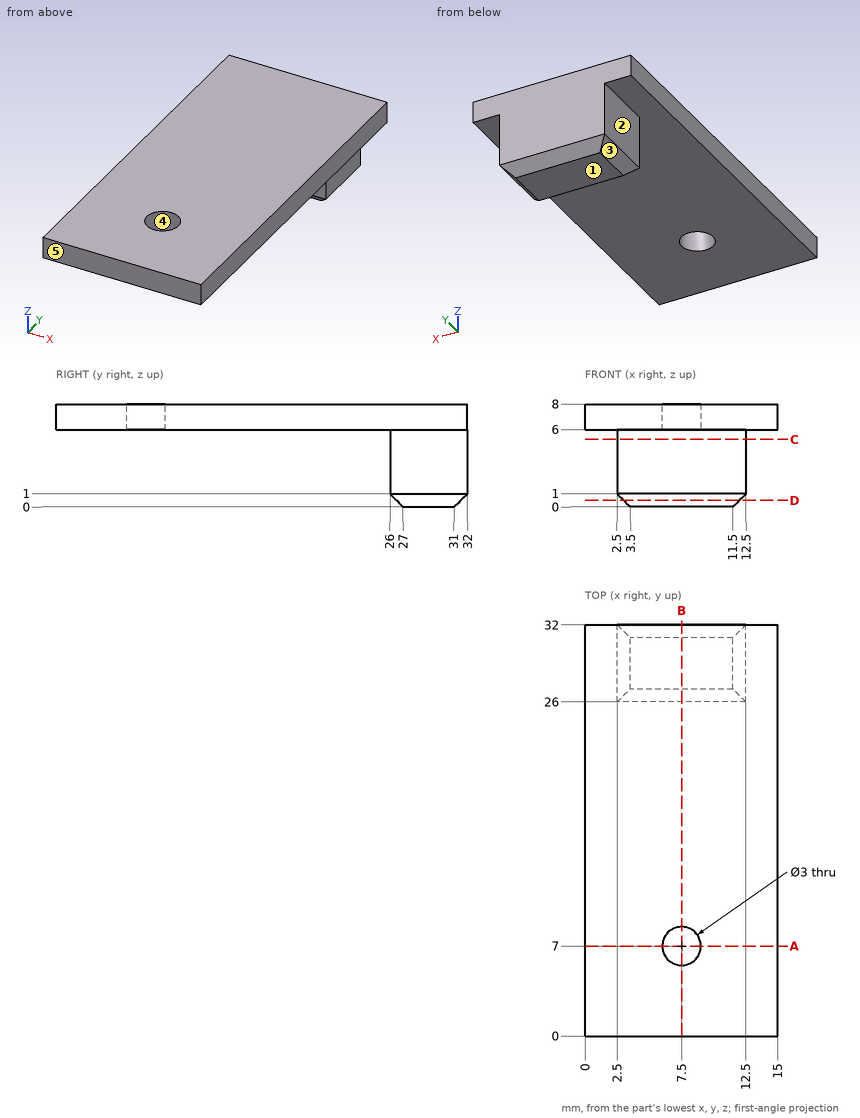
Here's the drawing with two shaded views (mm, measured from the low corner). I have some questions. A direction names the side the tool comes from. Give positions to 0.01 mm unless a question says otherwise; leave off trailing zeros. Write each loop counter-clockwise with the first axis right and the second up, starting at its lowest first coordinate (ties: lowest second). Pieces come first, ordered by that corner, then holes. Notation, with made-up numbers: (28.25, 50.25) - (47.25, 50.25) arc R28 ccw to (47.25, 70.25) - close; hole circle Ø5 at (-39.75, 50.25). An arc over 180 degrees is marked (long way). One line per item, written item: value. Start each with the question number.
Item 1: Please list where these lines run through material, in increasing order: line 1 (Y direction, x = 7.5, z = 6.85); line 2 (Y direction, x = 10.5, z = 1.5); line 3 (Z direction, x = 5.5, y = 10). Write a range as from..to.
Item 2: Which directions (+Z, -Z, +X, -X, +Y, -Y) give clear straight access to the entire face, cutting with the end or side of a thin tool? Please do the marked faces 1 and 2.
Item 3: Imagine slicing it at B-B, the plane x = 7.5. List the corners of the cut face in (y, z) for me, and give its area (3 significant figures).
Item 4: If we mould it in two halves opening along X, with no side actions, what happens to the marked faces 3, 4 and 5? For each: +X half, -X half, draft (parallel to the pull), parting line (faces both ways), or undercut.
Item 5: Imagine slicing it at A-A, the plane y = 7. List the corners of the cut face in (x, z) for me.
Item 6: Imagine slicing it at C-C, the plane z = 5.25. List the corners of the cut face in (x, y) for me.
Item 7: Imagine slicing it at D-D, the plane z = 0.5. List the corners of the cut face in (x, y) for me.
Item 8: I'm going to push flat-ended pins straight in: pin 1 (7.5 mm diameter, centred on x = 9, y = 17.5, fed in from -Z); pin 2 (1.5 mm diameter, centred on x = 8, z = 4, fed in from -Y); pin 3 (2 mm diameter, centred on y = 25.5, z = 2, fed in from +X). Where does each tip first touch, or does it pass through?
Geometry says:
1. line 1: 0..5.5, 8.5..32
1. line 2: 26..32
1. line 3: 6..8
2. face 1: -Z, +X, -X, +Y, -Y
2. face 2: -Z, -X, +Y, -Y
3. outline: (0, 6) - (5.5, 6) - (5.5, 8) - (0, 8) - close; (8.5, 6) - (26, 6) - (26, 1) - (27, 0) - (31, 0) - (32, 1) - (32, 8) - (8.5, 8) - close
3. area: 93.0 mm^2
4. face 3: -X half
4. face 4: undercut
4. face 5: draft
5. outline: (0, 6) - (6, 6) - (6, 8) - (0, 8) - close; (9, 6) - (15, 6) - (15, 8) - (9, 8) - close
6. outline: (2.5, 26) - (12.5, 26) - (12.5, 32) - (2.5, 32) - close
7. outline: (3, 26.5) - (12, 26.5) - (12, 31.5) - (3, 31.5) - close
8. pin 1: z = 6
8. pin 2: y = 26
8. pin 3: x = 12.5
